CAD build for the part. Positions are in the model's coordinates, mm. Face numbers are marked on the shaded views. A direction names the side the tool comes from. Coordinates: 2 decimals unless noted, no trailing zeros. Order: outer loops, then holes, each group sorted by start corner. A loop starts at its lowest first (then second) coordinate and runs counter-clockwise, first axis right, second up. Notation, with made-up numbers: (62.5, 69.25) - (68.5, 69.25) arc R32 ccw to (68.5, 108.25) - close; hole circle Ø11 at (23, -26.75). An arc over 180 degrees is marked (long way). Return JSON: item names as keys, results as strings.
Autodesk Inventor part; units mm, degrees
ref_plane "YZ Plane" through (0, 0, 0) normal (1, 0, 0) x (0, 1, 0)
ref_plane "XY Plane" through (0, 0, 0) normal (0, 0, 1) x (1, 0, 0)
sketch "Sketch1" plane through (0, 0, 0) normal (0, 0, 1) x (1, 0, 0)
  circle A0 centre (71.5279, 0) radius 25.0279
  circle A1 centre (0, 0) radius 46.5
extrude "Extrusion1" add sketch "Sketch1" along normal mid plane 6 contours A0
sketch "Sketch2" plane through (71.5279, 0, -3) normal (0, 0, -1) x (-1, 0, 0)
  circle A0 centre (0, 0) radius 25.0279
  circle A1 centre (0, 0) radius 5.5
  point P0 (71.5279, 0)
  dimension "d2" = 11
extrude "Extrusion2" add sketch "Sketch2" along normal blind 6 contours A1
hole "Hole1" at (71.5279, 0, -9) direction (0, 0, 1) diameter 5.5 end through all
ref_plane "Work Plane1" through (71.5279, -5.5, -3) normal (0, 1, 0) x (-1, 0, 0)
sketch "Sketch3" plane through (71.5279, -5.5, -3) normal (0, 1, 0) x (-1, 0, 0)
  line L0 (-5.5, -6) -> (5.5, -6)
  line L1 (5.5, 0) -> (-5.5, 0)
  point P0 (71.5279, 3)
  point P1 (0.0146, -3)
  dimension "d14" = 3
hole "Hole2" at (71.5134, -5.5, -6) direction (0, 1, 0) diameter 3.5 end through all
properties part number "drive_wheel"
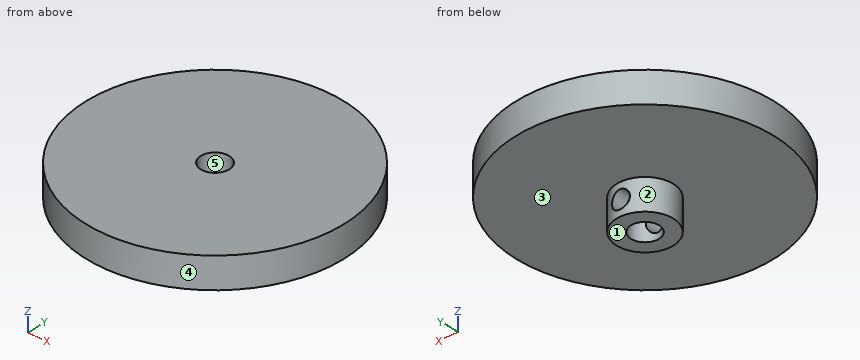
Item 1: Band-saw the part on A-A, the plane y = 0. List the corners of the cut face in (x, z).
Findings below:
{"outline": "(46.5, -3) - (66.03, -3) - (66.03, -9) - (68.78, -9) - (68.78, 3) - (46.5, 3) - close; (74.28, -9) - (77.03, -9) - (77.03, -3) - (96.56, -3) - (96.56, 3) - (74.28, 3) - close"}
Item 2: Band-saw the part on B-B, the plane z = -6. List the corners of the cut face in (x, y).
Findings below:
{"outline": "(69.76, -5.21) - (69.76, -2.11) arc R2.75 cw to (69.76, 2.11) - (69.76, 5.21) arc R5.5 ccw to start; (73.26, -5.22) arc R5.5 ccw to (73.26, 5.22) - (73.26, 2.13) arc R2.75 cw to (73.26, -2.13) - close"}
Item 3: Mould opens along Y. For the marked faces 3, 4 and 5 say: released by +Y, released by -Y, zero draft, split by the parting line, or undercut.
Findings below:
{"face 3": "zero draft", "face 4": "split by the parting line", "face 5": "undercut"}
Item 4: Drop flat-ended pins along their axis: P1, Ø6, axis at x = 68.5, z = 0, coming from the -Y side; P2, Ø2, axis at x = 71.51, z = -6, coming from the +Y side; P3, Ø3, axis at x = 87.5, y = -17.5, coming from the -Z side; P4, Ø1, axis at x = 90, z = -0.5, coming from the +Y side. Give the stop position or say it passes through.
Findings below:
{"P1": "stops at y = -25.03", "P2": "passes through", "P3": "stops at z = -3", "P4": "stops at y = 17.42"}
Item 5: Band-saw the part on C-C, the plane x = 57.5. List the corners of the cut face in (y, z), then the cut area to 3 significant figures.
Findings below:
{"outline": "(-20.73, -3) - (20.73, -3) - (20.73, 3) - (-20.73, 3) - close", "area": "249 mm²"}
Item 6: Which spindle directions (+Z, -Z, +X, -X, +Y, -Y) get a long thin tool onto all of the face, cutting with end or side? Do the marked faces 1 and 2. Say none if no direction does.
Findings below:
{"face 1": "-Z, +X, -X, +Y, -Y", "face 2": "-Z"}
Item 7: Band-saw the part on D-D, the plane z = -1.25. List the corners of the cut face in (x, y).
Findings below:
{"outline": "circle Ø50.06 at (71.53, 0); hole circle Ø5.5 at (71.53, 0)"}
Item 8: Wall check: L1, parallel to X at y = 0, z = -2.25; L2, parallel to Z at x = 84, y = -16; L3, parallel to Y at x = 72, z = 1.5. Give the ranges that are in metal, low to high. Write a range as [from, to].
Findings below:
{"L1": "x = [46.5, 68.78], [74.28, 96.56]", "L2": "z = [-3, 3]", "L3": "y = [-25.02, -2.71], [2.71, 25.02]"}
